from build123d import *

# Parameters (mm, degrees)
SKETCH1_R          = 3.4036
EXTRUDE1_DEPTH     = 190.5
CUT_EXTRUDE1_REACH = 197.079
CUT_EXTRUDE2_DEPTH = 3.048


with BuildPart() as part:
    # Sketch1 → Extrude1 (new, symmetric)
    with BuildSketch(Plane.XY):
        with BuildLine():
            Line((-20, 16.952), (-20, 4.7625))
            ThreePointArc((-20, 4.7625), (-19.776815367, 4.223684633), (-19.238, 4.0005))
            Line((-19.238, 4.0005), (-16.2662, 4.0005))
            ThreePointArc((-16.2662, 4.0005), (-15.727384633, 4.223684633), (-15.5042, 4.7625))
            Line((-15.5042, 4.7625), (-15.5042, 10.485558599))
            ThreePointArc((-15.5042, 10.485558599), (-15.033804775, 11.189554802), (-14.203384633, 11.024373966))
            Line((-14.203384633, 11.024373966), (-8.635059555, 5.456048889))
            ThreePointArc((-8.635059555, 5.456048889), (-7.985348265, 4.483687227), (-7.7572, 3.336708444))
            Line((-7.7572, 3.336708444), (-7.7572, -3.336708444))
            ThreePointArc((-7.7572, -3.336708444), (-7.985348265, -4.483687227), (-8.635059555, -5.456048889))
            Line((-8.635059555, -5.456048889), (-14.203384633, -11.024373966))
            ThreePointArc((-14.203384633, -11.024373966), (-15.033804775, -11.189554802), (-15.5042, -10.485558599))
            Line((-15.5042, -10.485558599), (-15.5042, -4.7625))
            ThreePointArc((-15.5042, -4.7625), (-15.727384633, -4.223684633), (-16.2662, -4.0005))
            Line((-16.2662, -4.0005), (-19.238, -4.0005))
            ThreePointArc((-19.238, -4.0005), (-19.776815367, -4.223684633), (-20, -4.7625))
            Line((-20, -4.7625), (-20, -16.952))
            ThreePointArc((-20, -16.952), (-19.107261469, -19.107261469), (-16.952, -20))
            Line((-16.952, -20), (-4.7625, -20))
            ThreePointArc((-4.7625, -20), (-4.223684633, -19.776815367), (-4.0005, -19.238))
            Line((-4.0005, -19.238), (-4.0005, -16.2662))
            ThreePointArc((-4.0005, -16.2662), (-4.223684633, -15.727384633), (-4.7625, -15.5042))
            Line((-4.7625, -15.5042), (-10.485558599, -15.5042))
            ThreePointArc((-10.485558599, -15.5042), (-11.189554802, -15.033804775), (-11.024373966, -14.203384633))
            Line((-11.024373966, -14.203384633), (-5.456048889, -8.635059555))
            ThreePointArc((-5.456048889, -8.635059555), (-4.483687227, -7.985348265), (-3.336708444, -7.7572))
            Line((-3.336708444, -7.7572), (3.336708444, -7.7572))
            ThreePointArc((3.336708444, -7.7572), (4.483687227, -7.985348265), (5.456048889, -8.635059555))
            Line((5.456048889, -8.635059555), (11.024373966, -14.203384633))
            ThreePointArc((11.024373966, -14.203384633), (11.189554802, -15.033804775), (10.485558599, -15.5042))
            Line((10.485558599, -15.5042), (4.7625, -15.5042))
            ThreePointArc((4.7625, -15.5042), (4.223684633, -15.727384633), (4.0005, -16.2662))
            Line((4.0005, -16.2662), (4.0005, -19.238))
            ThreePointArc((4.0005, -19.238), (4.223684633, -19.776815367), (4.7625, -20))
            Line((4.7625, -20), (16.952, -20))
            ThreePointArc((16.952, -20), (19.107261469, -19.107261469), (20, -16.952))
            Line((20, -16.952), (20, -4.7625))
            ThreePointArc((20, -4.7625), (19.776815367, -4.223684633), (19.238, -4.0005))
            Line((19.238, -4.0005), (16.2662, -4.0005))
            ThreePointArc((16.2662, -4.0005), (15.727384633, -4.223684633), (15.5042, -4.7625))
            Line((15.5042, -4.7625), (15.5042, -10.485558599))
            ThreePointArc((15.5042, -10.485558599), (15.033804775, -11.189554802), (14.203384633, -11.024373966))
            Line((14.203384633, -11.024373966), (8.635059555, -5.456048889))
            ThreePointArc((8.635059555, -5.456048889), (7.985348265, -4.483687227), (7.7572, -3.336708444))
            Line((7.7572, -3.336708444), (7.7572, 3.336708444))
            ThreePointArc((7.7572, 3.336708444), (7.985348265, 4.483687227), (8.635059555, 5.456048889))
            Line((8.635059555, 5.456048889), (14.203384633, 11.024373966))
            ThreePointArc((14.203384633, 11.024373966), (15.033804775, 11.189554802), (15.5042, 10.485558599))
            Line((15.5042, 10.485558599), (15.5042, 4.7625))
            ThreePointArc((15.5042, 4.7625), (15.727384633, 4.223684633), (16.2662, 4.0005))
            Line((16.2662, 4.0005), (19.238, 4.0005))
            ThreePointArc((19.238, 4.0005), (19.776815367, 4.223684633), (20, 4.7625))
            Line((20, 4.7625), (20, 16.952))
            ThreePointArc((20, 16.952), (19.107261469, 19.107261469), (16.952, 20))
            Line((16.952, 20), (4.7625, 20))
            ThreePointArc((4.7625, 20), (4.223684633, 19.776815367), (4.0005, 19.238))
            Line((4.0005, 19.238), (4.0005, 16.2662))
            ThreePointArc((4.0005, 16.2662), (4.223684633, 15.727384633), (4.7625, 15.5042))
            Line((4.7625, 15.5042), (10.485558599, 15.5042))
            ThreePointArc((10.485558599, 15.5042), (11.189554802, 15.033804775), (11.024373966, 14.203384633))
            Line((11.024373966, 14.203384633), (5.456048889, 8.635059555))
            ThreePointArc((5.456048889, 8.635059555), (4.483687227, 7.985348265), (3.336708444, 7.7572))
            Line((3.336708444, 7.7572), (-3.336708444, 7.7572))
            ThreePointArc((-3.336708444, 7.7572), (-4.483687227, 7.985348265), (-5.456048889, 8.635059555))
            Line((-5.456048889, 8.635059555), (-11.024373966, 14.203384633))
            ThreePointArc((-11.024373966, 14.203384633), (-11.189554802, 15.033804775), (-10.485558599, 15.5042))
            Line((-10.485558599, 15.5042), (-4.7625, 15.5042))
            ThreePointArc((-4.7625, 15.5042), (-4.223684633, 15.727384633), (-4.0005, 16.2662))
            Line((-4.0005, 16.2662), (-4.0005, 19.238))
            ThreePointArc((-4.0005, 19.238), (-4.223684633, 19.776815367), (-4.7625, 20))
            Line((-4.7625, 20), (-16.952, 20))
            ThreePointArc((-16.952, 20), (-19.107261469, 19.107261469), (-20, 16.952))
        make_face()
        Circle(SKETCH1_R, mode=Mode.SUBTRACT)
    extrude(amount=EXTRUDE1_DEPTH, both=True)

    # Cut-Extrude1: up to this face of the body (flat: up to its plane)
    cut_extrude1_end = Plane(part.part.faces().sort_by_distance((-10.85725, 20, 0))[0])
    # Sketch6 → Cut-Extrude1 (cut, up to the picked face)
    with BuildSketch(Plane(origin=(0, -16.952, 0), x_dir=(-1, 0, 0), z_dir=(0, -1, 0)), mode=Mode.PRIVATE) as cut_extrude1_sk1:
        Polygon((-20, -93.69431704), (20, -133.69431704), (20, -190.5), (-20, -190.5), align=None)
    cut_extrude1_tool1 = split(extrude(cut_extrude1_sk1.sketch, amount=-CUT_EXTRUDE1_REACH, mode=Mode.PRIVATE), bisect_by=cut_extrude1_end, keep=Keep.BOTH, mode=Mode.PRIVATE)
    add(cut_extrude1_tool1.solids().sort_by(Axis((1.735983, -16.952, 151.229167), (0, 1, 0)))[0], mode=Mode.SUBTRACT)

    # Sketch7 → Cut-Extrude2 (cut)
    with BuildSketch(Plane(origin=(0, -16.952, 0), x_dir=(1, 0, 0), z_dir=(0, 1, 0))):
        Polygon((-20, -133.69431704), (20, -93.69431704), (20, -190.5), (-20, -190.5), align=None)
    extrude(amount=-CUT_EXTRUDE2_DEPTH, mode=Mode.SUBTRACT)


solid = part.part
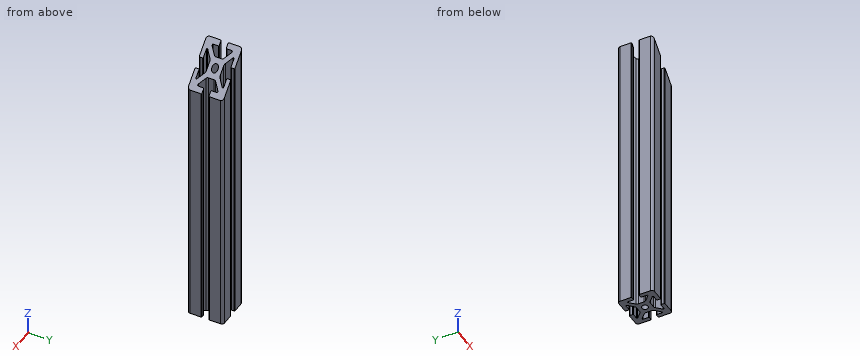
The listing builds one solid part. Answer for the finished solid, in the listing's coordinates (mm). Round coordinates to 2 decimals unless told otherwise and drop trailing zeros. Write each loop counter-clockwise with the first axis right and the second up, starting at its lowest first coordinate (ties: lowest second). Pieces come first, ordered by that corner, then holes. Notation, with made-up numbers: (82, 86) - (89, 86) arc R19 cw to (89, 91) - close; hole circle Ø9 at (-30, 26). An arc over 180 degrees is marked (long way). Use a Markdown table: item, result. Add a question column.
1. The part is cut by section A-A (x = 0). Write down the section's boundary in (y, z).
2. Consider line 1 (Y direction, x = 0, z = 37); line 2 (Y direction, x = -5, z = -3); line 3 (X direction, y = -15, z = 55). Determine where each line is inside the solid, lowest interval first.
3. Flat-ended cylindrical pins translate along their axes: P1, Ø3.5, axis at x = 18, z = 18.5, coming from the +Y side; P2, Ø0.9, axis at x = 18.5, z = 9, coming from the -Y side; P3, Ø4, axis at x = -8.5, y = -15.5, coming from the +Z side; P4, Ø1.5, axis at x = 1.5, z = -90.5, coming from the +Y side. Find the tip coordinate at first contact, or state that the pin passes through.
Reported:
| question | item | result |
|---|---|---|
| 1 | outline | (-7.76, -190.5) - (-3.4, -190.5) - (-3.4, 113.69) - (-7.76, 113.69) - close; (3.4, -190.5) - (7.76, -190.5) - (7.76, 113.69) - (3.4, 113.69) - close |
| 2 | line 1 | -7.76 to -3.4, 3.4 to 7.76 |
| 2 | line 2 | -20 to -15.5, -8.26 to 8.26, 15.5 to 20 |
| 2 | line 3 | -20 to -11.2, 11.2 to 20 |
| 3 | P1 | y = 20 |
| 3 | P2 | y = -19.8 |
| 3 | P3 | z = 124.19 |
| 3 | P4 | y = 7.76 |
